```python
from build123d import *

# Parameters (mm, degrees)
F1_DEPTH = 4
F2_DEPTH = 1
F3_DEPTH = 4


with BuildPart() as f1:
    # F0 (on Top) → F1 (new body)
    with BuildSketch(Plane.XY):
        with BuildLine():
            ThreePointArc((-1.5508525785, 7.9438418354), (-0.8117387783, 12.8375466645), (2.5605860204, 9.2151080362))
            ThreePointArc((2.5605860204, 9.2151080362), (3.7184283285, 7.9559790876), (5.2833155314, 8.6467269154))
            ThreePointArc((5.2833155314, 8.6467269154), (0.6891933533, 15.6793977841), (-5.5065598875, 10.00691509))
            Line((-5.5065598875, 10.00691509), (-5.4662271831, 9.5160487318))
            ThreePointArc((-5.4662271831, 9.5160487318), (-5.1890353006, 8.3580166056), (-4.6695398419, 7.2865698204))
            ThreePointArc((-4.6695398419, 7.2865698204), (-3.0526487171, 5.624718363), (-0.8952786583, 4.7751057418))
            Line((-0.8952786583, 4.7751057418), (-0.5786401844, 4.6951146522))
            Line((-0.5786401844, 4.6951146522), (1.5938929177, 4.1462764523))
            ThreePointArc((1.5938929177, 4.1462764523), (2.6825813347, 3.2735631577), (3.2693851036, 2.0076515096))
            ThreePointArc((3.2693851036, 2.0076515096), (3.3114958995, 1.7472962445), (3.3309836872, 1.4842783567))
            Line((3.3309836872, 1.4842783567), (3.4477516729, -0.9928926231))
            Line((3.4477516729, -0.9928926231), (3.9091161415, -10.7804954964))
            ThreePointArc((3.9091161415, -10.7804954964), (2.9687698725, -12.8820847985), (0.7233424694, -13.3909899741))
            ThreePointArc((0.7233424694, -13.3909899741), (-3.8310752971, -10.860666841), (-6.6450210288, -6.4758104272))
            ThreePointArc((-6.6450210288, -6.4758104272), (-7.7820397087, -4.8140308867), (-9.2495143625, -3.4353210333))
            ThreePointArc((-9.2495143625, -3.4353210333), (-9.2784237273, -3.4136155218), (-9.3074170873, -3.3920223359))
            ThreePointArc((-9.3074170873, -3.3920223359), (-11.2022703258, -4.1244357737), (-9.8017050698, -5.5959367772))
            ThreePointArc((-9.8017050698, -5.5959367772), (-8.7259718037, -6.0249943061), (-8.2120165113, -7.0628490071))
            ThreePointArc((-8.2120165113, -7.0628490071), (-5.7280471213, -11.5611556114), (-1.7350801949, -14.7955151093))
            ThreePointArc((-1.7350801949, -14.7955151093), (-1.4700198659, -14.9324899814), (-1.201978699, -15.0635358758))
            ThreePointArc((-1.201978699, -15.0635358758), (3.8524766741, -14.675655203), (6.3695942874, -10.2754177713))
            Line((6.3695942874, -10.2754177713), (5.7489675473, 1.5311539041))
            ThreePointArc((5.7489675473, 1.5311539041), (5.1595327201, 4.0189158193), (3.4136745307, 5.8866341986))
            add(Edge.make_bspline(
                [(-1.3902529619, 7.8420158064), (0.0180558581, 6.9514744016), (0.5184174589, 6.7699007224), (2.976767486, 6.2503702939), (3.4136745307, 5.8866341986)],
                knots=[0.018384806, 0.018384806, 0.018384806, 0.018384806, 0.516913737, 1, 1, 1, 1], degree=3))
            ThreePointArc((-1.3902529619, 7.8420158064), (-1.4714338534, 7.8915391799), (-1.5508525785, 7.9438418354))
        make_face()
    extrude(amount=F1_DEPTH)

    # F0 (on Top) → F2 (join)
    with BuildSketch(Plane.XY):
        with BuildLine():
            ThreePointArc((-0.8952786583, 4.7751057418), (-3.0526487171, 5.624718363), (-4.6695398419, 7.2865698204))
            Line((-4.6695398419, 7.2865698204), (-3.9393737235, -1.599865865))
            Line((-3.9393737235, -1.599865865), (3.4477516729, -0.9928926231))
            Line((3.4477516729, -0.9928926231), (3.3309836872, 1.4842783567))
            ThreePointArc((3.3309836872, 1.4842783567), (3.3114958995, 1.7472962445), (3.2693851036, 2.0076515096))
            Line((3.2693851036, 2.0076515096), (-0.3569517285, 1.7655659467))
            Line((-0.3569517285, 1.7655659467), (-0.5786401844, 4.6951146522))
            Line((-0.5786401844, 4.6951146522), (-0.8952786583, 4.7751057418))
        make_face()
    extrude(amount=F2_DEPTH)

    # F0 (on Top) → F3 (join)
    with BuildSketch(Plane.XY):
        with BuildLine():
            ThreePointArc((-4.6695398419, 7.2865698204), (-5.1890353006, 8.3580166056), (-5.4662271831, 9.5160487318))
            Line((-5.4662271831, 9.5160487318), (-4.5487587385, -1.6499368166))
            Line((-4.5487587385, -1.6499368166), (-3.9393737235, -1.599865865))
            Line((-3.9393737235, -1.599865865), (-4.6695398419, 7.2865698204))
        make_face()
    extrude(amount=F3_DEPTH)


solid = f1.part
```
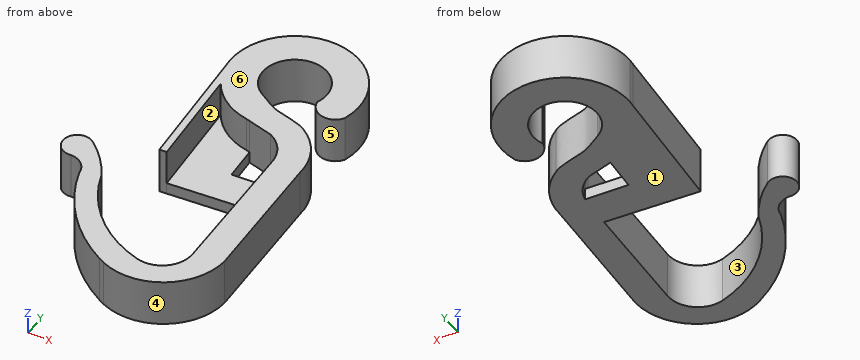
Can you work these out from the model? Positions are in its coordinate system, mm. Face numbers are marked on the shaded views. A direction names the side the tool comes from. Round coordinates to 2 decimals unless told otherwise and drop trailing zeros. Write item = value, one per line. Start each with the question number.
(1) Which directions (+Z, -Z, +X, -X, +Y, -Y) give clear straight access to the entire face, cutting with the end or side of a thin tool? Please do the marked faces 1, 2 and 3.
(2) I need wall thicknesses on line 1 along Y through (x, z) = (0, 1.25); line 2 along Y through (x, z) = (-2.5, 3.75); line 3 along Z through (x, y) = (-2.75, 5). Which ranges of each line are inside material? Lowest first, please.
(3) Suppose I cut it at A-A on x = 0. Give the number of separate pieces and of enclosed holes in the cut face, plus the area to 3 significant figures.
(4) I'm going to push flat-ended pins straight in: P1, Ø1, axis at x = -9, z = 1.5, coming from the -Y side; P2, Ø1, axis at y = -7, z = 2.5, coming from the +X side; P3, Ø2, axis at x = -3, y = 12, coming from the -Z side; P4, Ø2, axis at x = -9, z = 1, coming from the +Y side. Where does each tip first touch, or does it pass through?
(5) If we mould it in two halves opening along Y, with no side actions, what happens to the marked faces 4, 5 and 6? For each: released by +Y, released by -Y, zero draft, split by the parting line, or undercut.
Answer block:
q1.face_1 = -Z, +X, -X, +Y, -Y
q1.face_2 = +Z
q1.face_3 = +Z, -Z
q2.line_1 = -15.43 to -13.17, 4.55 to 7.02, 12.96 to 15.72
q2.line_2 = -14.36 to -11.92, 5.3 to 9.07, 11.35 to 15.12
q2.line_3 = 0 to 1
q3.separate_pieces = 4
q3.enclosed_holes = 0
q3.area = 33.0 mm²
q4.P1 = -6.28
q4.P2 = 6.22
q4.P3 = 0
q4.P4 = -3.17
q5.face_4 = released by -Y
q5.face_5 = undercut
q5.face_6 = zero draft
